Read the model definition and answer for the solid it produces. Units are mm, in the model's axes. Give positions to 0.01 mm unless a question says otherwise; leave off trailing zeros. Order: outer loops, then holes, each group sorted by start corner. A loop starts at its lowest first (then second) coordinate and runs counter-clockwise, first axis right, second up. Notation, with made-up numbers: M -10,89.5 L 13,89.5 A15 cw 13,109.5 Z; hole C 69,73 d7. An arc over 180 degrees is marked long. One line per item, written item: value.
from build123d import *

# Parameters (mm, degrees)
F0_R     = 1.45
F1_DEPTH = 2.5
F3_R     = 2.4
F3_R_2   = 1.45
F4_DEPTH = 1
F5_R     = 0.3


# Not quite as in the source:
# - a fillet or chamfer that OpenCascade refuses, or shapes differently, is made with other operations: its cross-section is extruded or revolved along the edge and cut away or added


with BuildPart() as f1:
    # F0 (on Top) → F1 (new body)
    with BuildSketch(Plane.XY):
        Polygon((-1.5886400056, -2.7494647235), (1.5867862946, -2.7505349641), (3.1754263002, -0.0010702406), (1.5886400056, 2.7494647235), (-1.5867862946, 2.7505349641), (-3.1754263002, 0.0010702406), align=None)
        Circle(F0_R, mode=Mode.SUBTRACT)
    extrude(amount=F1_DEPTH)

    # F3 (on offset) → F4 (join)
    with BuildSketch(Plane.XY.offset(2.5)):
        Circle(F3_R)
        Circle(F3_R_2, mode=Mode.SUBTRACT)
    extrude(amount=F4_DEPTH)

    # F5
    f5_edges = [f1.edges().sort_by_distance(p)[0] for p in [
        (-2.382033, -1.374197, 2.5),
        (-2.381106, 1.375803, 2.5),
        (0.000927, 2.75, 2.5),
        (2.382033, 1.374197, 2.5),
        (2.381106, -1.375803, 2.5),
        (-0.000927, -2.75, 2.5),
        (3.175426, -0.00107, 1.25),
        (1.58864, 2.749465, 1.25),
        (-1.586786, 2.750535, 1.25),
        (-3.175426, 0.00107, 1.25),
        (-1.58864, -2.749465, 1.25),
        (1.586786, -2.750535, 1.25),
    ]]
    fillet(f5_edges, radius=F5_R)

    # F6: fillet of radius 1 on 1 edges, made by hand

    # F6_s1 → F6_t2 (revolve, cut)
    with BuildSketch(Plane.XZ):
        with BuildLine():
            ThreePointArc((1.45, 3.5), (2.1245688373, 3.1904532198), (2.4, 2.5012507822))
            Line((2.4, 2.5012507822), (2.4, 3.5))
            Line((2.4, 3.5), (1.45, 3.5))
        make_face()
    revolve(axis=Axis((0, 0, 3.5), (0, 0, 1)), mode=Mode.SUBTRACT)


solid = f1.part
1) Determine the mould class of faces 1 (the face through (1.3, -1.2, 0)), 2 (the face through (-1.45, 0.06, 1.73)), 3 (the face through (-2.39, -1.36, 1.08)) for opening direction Y: +Y half, -Y half, draft (parallel to the pull), parting line (faces both ways), or undercut.
Reported:
face 1: draft
face 2: undercut
face 3: -Y half
2) Each of these flat-tipped pins is pushed along its axis until it touches: pin 1 Ø1.5 at (x, z) = (2.5, 1) entering from -Y; pin 2 Ø1.7 at (x, y) = (0, 0) entering from -Z. Where does it stop, or does it pass through?
Reported:
pin 1: stops at y = -2.47
pin 2: passes through
3) Consider probe 1 along Y at (x, z) = (0, 1.15); probe 2 along X at (y, z) = (1.25, 2.9); probe 3 along X at (y, z) = (-0.6, 2.2). Determine where each line is inside the solid, lowest interval first.
Reported:
probe 1: y = -2.75 to -1.45, 1.45 to 2.75
probe 2: x = -1.95 to -0.73, 0.73 to 1.95
probe 3: x = -2.83 to -1.32, 1.32 to 2.83
4) Find section B-B, the plane z = 3.1. Write down the section's boundary in (x, y), plus the area to 3 significant figures.
Reported:
outline: C 0,0 d4.4; hole C 0,0 d2.9
area: 8.61 mm^2
5) Find section A-A, the plane z = 2.05. Write down the section's boundary in (x, y), plus the area to 3 significant figures.
Reported:
outline: M -3.09,-0.15 L -1.68,-2.6 A0.3 ccw -1.42,-2.75 L 1.41,-2.75 A0.3 ccw 1.67,-2.6 L 3.09,-0.15 A0.3 ccw 3.09,0.15 L 1.68,2.6 A0.3 ccw 1.42,2.75 L -1.41,2.75 A0.3 ccw -1.67,2.6 L -3.09,0.15 A0.3 ccw Z; hole C 0,0 d2.9
area: 19.6 mm^2
